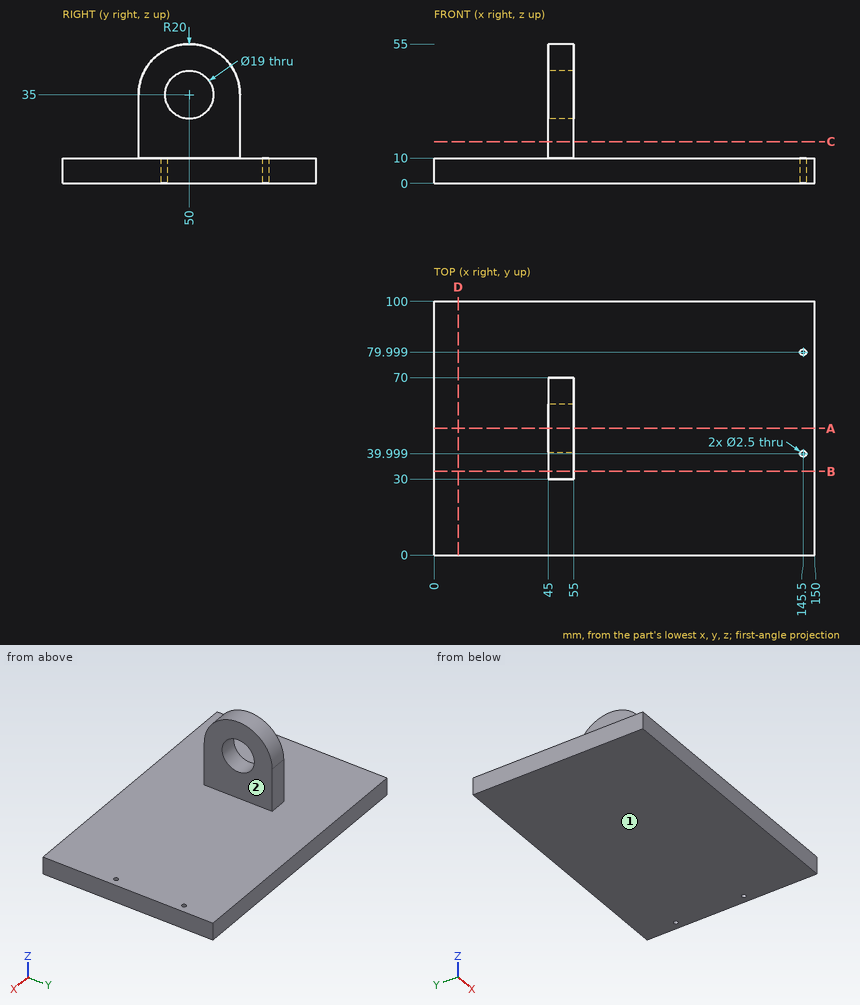
The drawing under review shows one solid part. Ordinate dimensions are in mm from its lowest x, y, z. A direction names the side the tool comes from. Give positions to 0.01 mm unless a question says otherwise; leave off trailing zeros. Loops run counter-clockwise (first coordinate to the right, second up) from the corner with the lowest first, then second, coordinate; pieces in that order, holes last. Notation, with made-up numbers: M 8.25,29 L 45.25,29 A27 ccw 45.25,63 Z; hole C 47,-37 d4. An arc over 180 degrees is marked long. One line per question, with ' | ' between items. Start each with the question number.
1. Add section B-B (y = 33). Write out the cut boundary in (x, z).
2. Add section A-A (y = 50). Write out the cut boundary in (x, z).
3. For the marked faces 1 and 2, list the 3-axis set-ups (+Z, -Z, +X, -X, +Y, -Y) from which the entire face can be reached by the end or side of a thin tool; tool diameter is ignored.
4. To check wall thickness, follow L1, parallel to Y at x = 145.5, z = 2.75; L2, parallel to Y at x = 145, z = 6 (1 decimal); L3, parallel to Z at x = 52.5, y = 50. State the ranges of each line that lie inside material, in increasing order.
5. Add section D-D (x = 9.5). Write out the cut boundary in (y, z), plus the area to 3 significant figures.
6. Add section C-C (z = 16.5). Write out the cut boundary in (x, y).
7. Insertion check: P1, Ø10, axis at y = 44, z = 35, coming from the +X side; P2, Ø6, axis at x = 80.5, y = 49, coming from the +Z side; P3, Ø22, axis at y = 50, z = 35, coming from the -X side. Each pin has a flat end and moves straight along its axis. Give the tip position at first contact, or say it passes through.
Worked out:
1) outline: M 0,0 L 150,0 L 150,10 L 55,10 L 55,45.54 L 45,45.54 L 45,10 L 0,10 Z
2) outline: M 0,0 L 150,0 L 150,10 L 55,10 L 55,25.5 L 45,25.5 L 45,10 L 0,10 Z; M 45,44.5 L 55,44.5 L 55,55 L 45,55 Z
3) face 1: -Z, +X, -X, +Y, -Y | face 2: +Z, +X, +Y, -Y
4) L1: y = 0 to 38.75, 41.25 to 78.75, 81.25 to 100 | L2: y = 0 to 38.9, 41.1 to 78.9, 81.1 to 100 | L3: z = 0 to 25.5, 44.5 to 55
5) outline: M 0,0 L 100,0 L 100,10 L 0,10 Z | area: 1,000 mm²
6) outline: M 45,30 L 55,30 L 55,70 L 45,70 Z
7) P1: stops at x = 55 | P2: stops at z = 10 | P3: stops at x = 45
